```python
from build123d import *


with BuildPart() as f1:
    # F0 (on Front) → F1 (revolve)
    with BuildSketch(Plane.XZ):
        with BuildLine():
            ThreePointArc((-30, -40), (-15.8113883008, -47.4341649025), (0, -50))
            Line((0, -50), (0, 50))
            ThreePointArc((0, 50), (-47.4341649025, 15.8113883008), (-30, -40))
        make_face()
        with BuildLine():
            Line((0, -56), (0, -50))
            ThreePointArc((0, -50), (-15.8113883008, -47.4341649025), (-30, -40))
            Line((-30, -40), (-30, -56))
            Line((-30, -56), (0, -56))
        make_face()
        Polygon((-60, -56), (-45, -56), (-55, -46), (-60, -46), align=None)
        Polygon((0, -156), (0, -56), (-30, -56), (-45, -56), (-60, -56), (-60, -156), align=None)
    revolve(axis=Axis((0, 0, -3), (0, 0, -1)))


solid = f1.part
```
Build history of the part. All positions in model axes, mm. A direction names the side the tool comes from. Round coordinates to 2 decimals unless told otherwise and drop trailing zeros. Write each loop counter-clockwise with the first axis right and the second up, starting at its lowest first coordinate (ties: lowest second). Pieces come first, ordered by that corner, then holes. Notation, with made-up numbers: (-21, -23) - (9, -23) arc R30 cw to (9, 1) - close; hole circle Ø4 at (83.25, 43.5). An arc over 180 degrees is marked (long way). Answer as CSV lines item,"result".
Q1. Tool access for faces 1 (the cylindrical face through (59.94, 2.64, -101.77)), 2 (the cylindrical face through (29.97, 1.32, -48.11)): list every direction of +Z, -Z, +X, -X, +Y, -Y with a clear straight run to the whole face (end or side of a thin tool).
Report:
face 1,"+Z, -Z"
face 2,"none"
Q2. Cut at C-C (z = -96.5). Write the cut outline in (x, y).
Report:
outline,"circle Ø120 at (0, 0)"
Q3. Drop flat-ended pins along their axis: pin 1 (12 mm diameter, centred on y = 32, z = -78.5, fed in from +X); pin 2 (1 mm diameter, centred on x = 21, z = -64, fed in from +Y); pin 3 (5 mm diameter, centred on x = -40, z = 6, fed in from +Y). Give the stop position or say it passes through.
Report:
pin 1,"stops at x = 54.07"
pin 2,"stops at y = 56.39"
pin 3,"stops at y = 32.56"
Q4. Drill centre lines: probe 1 along Z at (x, y) = (-18, 33); probe 2 along Z at (x, y) = (19, 27.5); probe 3 along Y at (x, z) = (-32.5, -95). Where is each one in solid material? Low to high. Write a range as [from, to].
Report:
probe 1,"z = [-156, -56], [-32.97, 32.97]"
probe 2,"z = [-156, -56], [-37.19, 37.19]"
probe 3,"y = [-50.44, 50.44]"
Q5. Cut at A-A (x = 0). Write the cut outline in (y, z).
Report:
outline,"(-60, -156) - (60, -156) - (60, -46) - (55, -46) - (45, -56) - (30, -56) - (30, -40) arc R50 ccw (long way) to (-30, -40) - (-30, -56) - (-45, -56) - (-55, -46) - (-60, -46) - close"
Q6. Pull direction Z, two halves, no side cores. Call faces 3 (the conical face through (9.891, -44.541, -55.374)), 4 (the flat face through (1, 1, -156)), 5 (the flat face through (26, -49, -46)): +Z half, -Z half, draft (parallel to the pull), parting line (faces both ways), or undercut.
Report:
face 3,"undercut"
face 4,"-Z half"
face 5,"+Z half"
